Source: CAD feature listing. Evaluate the final solid. Frame: model axes, mm. Face numbers are marked on the shaded views. A direction names the side the tool comes from. Give positions to 0.01 mm unless a question says otherwise; leave off trailing zeros. Write each loop counter-clockwise with the first axis right and the second up, starting at its lowest first coordinate (ties: lowest second). Pieces come first, ordered by that corner, then holes. Notation, with made-up numbers: (87, -33.5) -> (96, -33.5) arc R27 cw to (96, 0.5) -> close; hole circle Ø10 at (51.25, 53.25). An arc over 180 degrees is marked (long way). Answer as a JSON object with one key per item and string values. Group by question number.
Item 1: First-contact query: pin 1 Ø5 at (y, z) = (-15.875, 0) entering from -X; pin 2 Ø2 at (x, z) = (-6, -2.5) entering from +Y; pin 3 Ø4 at (x, z) = (-9, 6.5) entering from +Y; pin 4 Ø3 at (x, y) = (-2, 1) entering from -Z (3 decimals). Flat tips, straight axial feed; report the tip coordinate or a pass-through.
Item 2: Pull-direction query (Y, two-part tool) for the marked faces 1, 2 and 3; classes: pulls with the +Y half, pulls with the -Y half, needs draft (parallel to the pull), parting line crosses it, or undercut.
Item 3: Ray query, probe 1 along Z at (x, y) = (-1.8, 0) (1 decimal); probe 2 along Z at (x, y) = (-4, 0) (3 decimals); probe 3 along Y at (x, z) = (-6.25, 9). Return the intervals inside material, ascending. Write a range as from..to.
Item 4: Access query for the marked faces 4 and 5. Directions: +Z, -Z, +X, -X, +Y, -Y. A direction counts if a zero-diameter tool reaches every point of the face in a straight line with its end or side. Return the directions, or none.
Item 5: Section query C-C on z = 13. Return the cut outline in (x, y), plus the area to 3 significant figures.
Item 6: Section query D-D on x = -12.5. Return the cut outline in (y, z), plus the area to 3 significant figures.
Item 7: Section query A-A on z = 0. Give the number of separate pieces and of enclosed holes in the cut face, plus the area to 3 significant figures.
from build123d import *

# Parameters (mm, degrees)
SKETCH2_R          = 3.96875
CUT_EXTRUDE1_DEPTH = 33.341392209
SKETCH4_R          = 2.5
CUT_EXTRUDE2_DEPTH = 9.7155
SKETCH5_R          = 1.5875
CUT_EXTRUDE3_DEPTH = 2.38125
SKETCH6_W          = 1.1303
SKETCH6_H          = 22.225


with BuildPart() as part:
    # Sketch1 → Revolve1 (revolve)
    with BuildSketch(Plane.XY):
        Polygon((0, 0), (0, 22.225), (-6.858, 22.225), (-6.858, 6.35), (-14.478, 6.35), (-14.478, 0), align=None)
    revolve(axis=Axis((0, 0, 0), (-1, 0, 0)))

    # Sketch2 → Cut-Extrude1 (cut, through all)
    with BuildSketch(Plane.ZY.offset(6.858)):
        with Locations(Location((0, 15.875, 0), (0, 0, 270))):
            Circle(SKETCH2_R)
        with Locations(Location((11.225320151, 11.225320151, 0), (0, 0, 270))):
            Circle(SKETCH2_R)
        with Locations(Location((15.875, 0, 0), (0, 0, 270))):
            Circle(SKETCH2_R)
        with Locations(Location((11.225320151, -11.225320151, 0), (0, 0, 270))):
            Circle(SKETCH2_R)
        with Locations(Location((0, -15.875, 0), (0, 0, 270))):
            Circle(SKETCH2_R)
        with Locations(Location((-11.225320151, -11.225320151, 0), (0, 0, 270))):
            Circle(SKETCH2_R)
        with Locations(Location((-15.875, 0, 0), (0, 0, 270))):
            Circle(SKETCH2_R)
        with Locations(Location((-11.225320151, 11.225320151, 0), (0, 0, 270))):
            Circle(SKETCH2_R)
    extrude(amount=-CUT_EXTRUDE1_DEPTH, mode=Mode.SUBTRACT)

    # Sketch4 → Cut-Extrude2 (cut)
    with BuildSketch(Plane.ZY.offset(14.478)):
        with Locations(Location((0, 0, 0), (0, 0, 270))):
            Circle(SKETCH4_R)
    extrude(amount=-CUT_EXTRUDE2_DEPTH, mode=Mode.SUBTRACT)

    # Sketch5 → Cut-Extrude3 (cut)
    with BuildSketch(Plane(origin=(0, 0, 0), x_dir=(0, 0, -1), z_dir=(1, 0, 0))):
        with Locations(Location((0, 0, 0), (0, 0, 90))):
            Circle(SKETCH5_R)
        with Locations(Location((-17.599905094, 7.290119387, 0), (0, 0, 90))):
            Circle(SKETCH5_R)
        with Locations(Location((7.290119387, 17.599905094, 0), (0, 0, 90))):
            Circle(SKETCH5_R)
        with Locations(Location((17.599905094, -7.290119387, 0), (0, 0, 90))):
            Circle(SKETCH5_R)
        with Locations(Location((-7.290119387, -17.599905094, 0), (0, 0, 90))):
            Circle(SKETCH5_R)
    extrude(amount=-CUT_EXTRUDE3_DEPTH, mode=Mode.SUBTRACT)

    # Sketch6 → #4-40 Tapped Hole1 (revolve, cut)
    with BuildSketch(Plane.YZ.offset(-10.668)):
        with Locations((0.56515, 11.1125)):
            Rectangle(SKETCH6_W, SKETCH6_H)
    revolve(axis=Axis((-10.668, 0, -6.35), (0, 0, 1)), mode=Mode.SUBTRACT)


solid = part.part
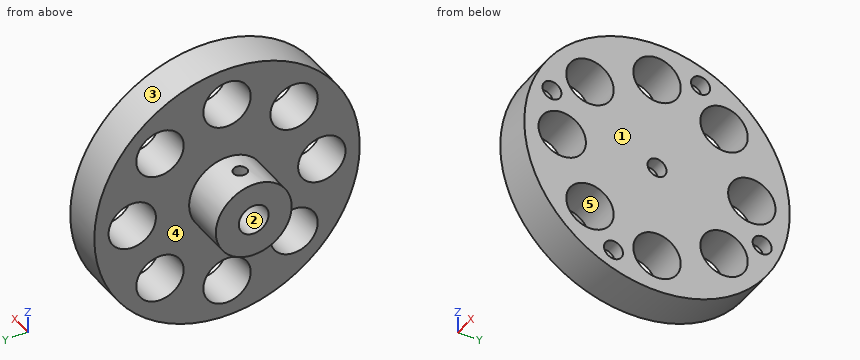
Worked answers:
{
 "1": {"pin 1": "through", "pin 2": "y = 22.17", "pin 3": "y = 4.48", "pin 4": "z = -22.225"},
 "2": {"face 1": "needs draft", "face 2": "undercut", "face 3": "parting line crosses it"},
 "3": {"probe 1": "-22.2..-19.8, -11.9..-1.6, 1.6..11.9, 19.8..22.2", "probe 2": "-22.225..-19.844, -11.906..11.906, 19.844..22.225", "probe 3": "-20.32..-14.51, -7.94..7.94, 14.51..20.32"},
 "4": {"face 4": "-X", "face 5": "+X, -X"},
 "5": {"outline": "(-6.86, -18.03) -> (0, -18.03) -> (0, -14.78) -> (-6.86, -14.78) -> close; (-6.86, -7.68) -> (0, -7.68) -> (0, -2.74) -> (-6.86, -2.74) -> close; (-6.86, 2.74) -> (0, 2.74) -> (0, 7.68) -> (-6.86, 7.68) -> close; (-6.86, 14.78) -> (0, 14.78) -> (0, 18.03) -> (-6.86, 18.03) -> close", "area": "112 mm^2"},
 "6": {"outline": "circle Ø12.7 at (0, 0); hole circle Ø5 at (0, 0)", "area": "107 mm^2"},
 "7": {"separate pieces": "3", "enclosed holes": "0", "area": "237 mm^2"}
}
